```python
from build123d import *

# Parameters (mm, degrees)
SKETCH1_R           = 12.7
SKETCH1_R_2         = 1.1
BOSS_EXTRUDE1_DEPTH = 4
SKETCH2_R           = 13.97
CUT_EXTRUDE1_DEPTH  = 3.175


with BuildPart() as part:
    # Sketch1 → Boss-Extrude1 (new body)
    with BuildSketch(Plane.XY):
        Polygon((-44, 19.9319), (-44, 5.39), (-49.715, 5.39), (-49.715, -5.39), (-44, -5.39), (-44, -19.9319), (44, -19.9319), (44, -5.39), (49.715, -5.39), (49.715, 5.39), (44, 5.39), (44, 19.9319), align=None)
        Circle(SKETCH1_R, mode=Mode.SUBTRACT)
        with Locations((-46.3876, 0)):
            Circle(SKETCH1_R_2, mode=Mode.SUBTRACT)
        with Locations(Location((46.3876, 0, 0), (0, 0, 180))):
            Circle(SKETCH1_R_2, mode=Mode.SUBTRACT)
    extrude(amount=BOSS_EXTRUDE1_DEPTH)

    # Sketch2 → Cut-Extrude1 (cut)
    with BuildSketch(Plane.XY.offset(4)):
        Circle(SKETCH2_R)
    extrude(amount=-CUT_EXTRUDE1_DEPTH, mode=Mode.SUBTRACT)


solid = part.part
```
Could you check a few things on this model? Use its own coordinates, in mm. A direction names the side the tool comes from. Round coordinates to 2 decimals unless told otherwise and drop trailing zeros. Loops run counter-clockwise (first coordinate to the right, second up) from the corner with the lowest first, then second, coordinate; pieces in that order, holes last.
Q1. For P1, Ø10, axis at x = -31.5, y = -10, coming from the -Z side; P2, Ø1.2, axis at x = -46, z = 2, coming from the +Y side; P3, Ø2, axis at y = 10.5, z = 2, coming from the -X side, each with a flat end and sliding along its axis, tell me the tip position at first contact or that it passes through.
Q2. I want a section at C-C (z = 1.55). Write out the boundary of the cut face in (x, y) (3 decimals), and give its area (3 significant figures).
Q3. I want a section at B-B (x = 0). Write out the boundary of the cut face in (y, z) (3 decimals).
Q4. Please list where these lines run through material, in increasing order: L1, parallel to Y at x = 0, z = 3.45; L2, parallel to X at y = 1, z = 3.1 (3 decimals); L3, parallel to Y at x = 0, z = 0.5.
Q5. I want a section at D-D (y = 9). Write out the boundary of the cut face in (x, z) (3 decimals).
Q6. I want a section at A-A (y = 0). Write out the boundary of the cut face in (x, z) (3 decimals), and give its area (3 significant figures).
Q7. On a 3-axis mill with a long thin cutter (end or side, diameter ignored), from which of +Z, -Z, +X, -X, +Y, -Y can I reach the whole of each face in a straight line? I mean faces 1 (the cylindrical face through (-1.82, 13.85, 2.43)), 2 (the flat face through (-47, -5.39, 2)), 3 (the flat face through (-47, 5.39, 2)), 4 (the flat face through (44, -13, 2)), 5 (the flat face through (44, 13, 2)). Say none if no direction works.
Q8. Thinking about a two-plate mould opening in Y: for faces 6 (the flat face through (-44, 13, 2)), 7 (the flat face through (47, -5.39, 2)), 8 (the flat face through (6.14, -11.32, 0.825)), 9 (the flat face through (1, 19.932, 2)), which applies, pulls with the +Y half, pulls with the -Y half, needs draft (parallel to the pull), parting line crosses it, or undercut?
Answer below:
1. P1: stops at z = 0
1. P2: stops at y = 5.39
1. P3: stops at x = -44
2. outline: (-49.715, -5.39) - (-44, -5.39) - (-44, -19.932) - (44, -19.932) - (44, -5.39) - (49.715, -5.39) - (49.715, 5.39) - (44, 5.39) - (44, 19.932) - (-44, 19.932) - (-44, 5.39) - (-49.715, 5.39) - close; hole circle Ø2.2 at (-46.388, 0); hole circle Ø27.94 at (0, 0); hole circle Ø2.2 at (46.388, 0)
2. area: 3,010 mm2
3. outline: (-19.932, 0) - (-12.7, 0) - (-12.7, 0.825) - (-13.97, 0.825) - (-13.97, 4) - (-19.932, 4) - close; (12.7, 0) - (19.932, 0) - (19.932, 4) - (13.97, 4) - (13.97, 0.825) - (12.7, 0.825) - close
4. L1: y = -19.93 to -13.97, 13.97 to 19.93
4. L2: x = -49.715 to -46.846, -45.929 to -13.934, 13.934 to 45.929, 46.846 to 49.715
4. L3: y = -19.93 to -12.7, 12.7 to 19.93
5. outline: (-44, 0) - (-8.96, 0) - (-8.96, 0.825) - (-10.685, 0.825) - (-10.685, 4) - (-44, 4) - close; (8.96, 0) - (44, 0) - (44, 4) - (10.685, 4) - (10.685, 0.825) - (8.96, 0.825) - close
6. outline: (-49.715, 0) - (-47.488, 0) - (-47.488, 4) - (-49.715, 4) - close; (-45.288, 0) - (-12.7, 0) - (-12.7, 0.825) - (-13.97, 0.825) - (-13.97, 4) - (-45.288, 4) - close; (12.7, 0) - (45.288, 0) - (45.288, 4) - (13.97, 4) - (13.97, 0.825) - (12.7, 0.825) - close; (47.488, 0) - (49.715, 0) - (49.715, 4) - (47.488, 4) - close
6. area: 270 mm2
7. face 1: +Z
7. face 2: +Z, -Z, -X, -Y
7. face 3: +Z, -Z, -X, +Y
7. face 4: +Z, -Z, +X, -Y
7. face 5: +Z, -Z, +X, +Y
8. face 6: needs draft
8. face 7: pulls with the -Y half
8. face 8: undercut
8. face 9: pulls with the +Y half
